Geometry check sheet. Reference: the model listing, model coordinates, mm. Coordinates: 2 decimals unless noted, no trailing zeros. Loops run counter-clockwise (first coordinate to the right, second up) from the corner with the lowest first, then second, coordinate; pieces in that order, holes last.
from build123d import *

# Parameters (mm, degrees)
SKETCH_1_R      = 50
SKETCH_1_R_2    = 2
SKETCH_1_R_3    = 26.5
EXTRUDE_1_DEPTH = 4


with BuildPart() as part:
    # 草图1 → 凸台-拉伸1 (new body)
    with BuildSketch(Plane.XY):
        with Locations((0, -21.854285714)):
            Circle(SKETCH_1_R)
        with Locations((-20, 18.145714286)):
            Circle(SKETCH_1_R_2, mode=Mode.SUBTRACT)
        with Locations((20, 18.145714286)):
            Circle(SKETCH_1_R_2, mode=Mode.SUBTRACT)
        with Locations(Location((20, -61.854285714, 0), (0, 0, 180))):
            Circle(SKETCH_1_R_2, mode=Mode.SUBTRACT)
        with Locations(Location((-20, -61.854285714, 0), (0, 0, 180))):
            Circle(SKETCH_1_R_2, mode=Mode.SUBTRACT)
        with Locations((0, -21.854285714)):
            Circle(SKETCH_1_R_3, mode=Mode.SUBTRACT)
    extrude(amount=EXTRUDE_1_DEPTH)


solid = part.part
(1) Sectioned sample at C-C on x = -20. Record the cut outline in (y, z).
Findings:
outline: (-67.68, 0) - (-63.85, 0) - (-63.85, 4) - (-67.68, 4) - close; (-59.85, 0) - (-39.24, 0) - (-39.24, 4) - (-59.85, 4) - close; (-4.47, 0) - (16.15, 0) - (16.15, 4) - (-4.47, 4) - close; (20.15, 0) - (23.97, 0) - (23.97, 4) - (20.15, 4) - close
(2) Sectioned sample at B-B on y = 1.5. Record the cut outline in (x, z).
Findings:
outline: (-44.21, 0) - (-12.52, 0) - (-12.52, 4) - (-44.21, 4) - close; (12.52, 0) - (44.21, 0) - (44.21, 4) - (12.52, 4) - close
(3) Sectioned sample at D-D on z = 1.4. Record the cut outline in (x, y), and give its area (3 significant figures).
Findings:
outline: circle Ø100 at (0, -21.85); hole circle Ø53 at (0, -21.85); hole circle Ø4 at (-20, -61.85); hole circle Ø4 at (-20, 18.15); hole circle Ø4 at (20, -61.85); hole circle Ø4 at (20, 18.15)
area: 5,600 mm2
(4) Gauge pin test, flat end, axial feed: pin 1 Ø2 at (y, z) = (-34.5, 1) entering from +X. Record the tip position at first contact, or that the pin passes through.
Findings:
pin 1: stops at x = 48.62
(5) Scan lines: L1, parallel to Y at x = 0, z = 1.25; L2, parallel to Y at x = 21.5, z = 2.45; L3, parallel to X at y = -62.5, z = 1.5. Record each from-to range of solid material in increasing order.
Findings:
L1: y = -71.85 to -48.35, 4.65 to 28.15
L2: y = -67 to -63.18, -60.53 to -37.35, -6.36 to 16.82, 19.47 to 23.29
L3: x = -29.12 to -21.89, -18.11 to 18.11, 21.89 to 29.12
(6) Sectioned sample at A-A on x = 0. Record the cut outline in (y, z), and give its area (3 significant figures).
Findings:
outline: (-71.85, 0) - (-48.35, 0) - (-48.35, 4) - (-71.85, 4) - close; (4.65, 0) - (28.15, 0) - (28.15, 4) - (4.65, 4) - close
area: 188 mm2
(7) Draft check along Y on faces 1 (the flat face through (22, -43, 0)), 2 (the cylindrical face through (-19.74, -63.837, 1.972)), 3 (the cylindrical face through (23.1, -66.2, 2)). Enter one of: +Y half, -Y half, draft (parallel to the pull), parting line (faces both ways), or undercut.
Findings:
face 1: draft
face 2: undercut
face 3: parting line
